```python
from build123d import *

# Parameters (mm, degrees)
SKETCH1_W                      = 50
SKETCH1_H                      = 35
SKETCH1_R                      = 8.5
BOSS_EXTRUDE1_DEPTH            = 8
F_3_0MM_DOWEL_HOLE1_AT_2_COUNT = 2
F_3_0MM_DOWEL_HOLE1_AT_2_PITCH = 40.311288741
M5X0_8_TAPPED_HOLE1_AT_2_COUNT = 2
M5X0_8_TAPPED_HOLE1_AT_2_PITCH = 40.311288741
SKETCH6_R                      = 11.5
CUT_EXTRUDE1_DEPTH             = 1.5
CHAMFER1_SIZE                  = 1
CHAMFER2_SIZE                  = 0.2


with BuildPart() as part:
    # Sketch1 → Boss-Extrude1 (new body)
    with BuildSketch(Plane(origin=(0, 0, 0), x_dir=(1, 0, 0), z_dir=(0, 1, 0))):
        Rectangle(SKETCH1_W, SKETCH1_H)
        with Locations(Location((0, 0, 0), (0, 0, 270))):
            Circle(SKETCH1_R, mode=Mode.SUBTRACT)
    extrude(amount=BOSS_EXTRUDE1_DEPTH)

    # Sketch3 → Ø3.0mm Dowel Hole1 (revolve, cut)
    with BuildSketch(Plane(origin=(-17.5, 8, -10), x_dir=(0, 0, 1), z_dir=(1, 0, 0))):
        Polygon((0, 0), (0, 8), (1.75, 8), (1.5, 7.75), (1.5, 0.25), (1.75, 0), align=None)
    f_3_0mm_dowel_hole1 = revolve(axis=Axis((-17.5, 14.35, -10), (0, -1, 0)), mode=Mode.SUBTRACT)

    # Ø3.0mm Dowel Hole1 at 2: Ø3.0mm Dowel Hole1 ×2
    with Locations(*[Vector(0.8682431421244593, 0, 0.49613893835683387) * (i * F_3_0MM_DOWEL_HOLE1_AT_2_PITCH) for i in range(1, F_3_0MM_DOWEL_HOLE1_AT_2_COUNT)]):
        add(f_3_0mm_dowel_hole1, mode=Mode.SUBTRACT)

    # Sketch5 → M5x0.8 Tapped Hole1 (revolve, cut)
    with BuildSketch(Plane(origin=(17.5, 8, -10), x_dir=(0, 0, 1), z_dir=(1, 0, 0))):
        Polygon((0, 0), (0, 8), (3, 8), (2.1, 7.1), (2.1, 0.9), (3, 0), align=None)
    m5x0_8_tapped_hole1 = revolve(axis=Axis((17.5, 14.35, -10), (0, -1, 0)), mode=Mode.SUBTRACT)

    # M5x0.8 Tapped Hole1 at 2: M5x0.8 Tapped Hole1 ×2
    with Locations(*[Vector(-0.8682431421244593, 0, 0.49613893835683387) * (i * M5X0_8_TAPPED_HOLE1_AT_2_PITCH) for i in range(1, M5X0_8_TAPPED_HOLE1_AT_2_COUNT)]):
        add(m5x0_8_tapped_hole1, mode=Mode.SUBTRACT)

    # Sketch6 → Cut-Extrude1 (cut)
    with BuildSketch(Plane(origin=(0, 8, 0), x_dir=(1, 0, 0), z_dir=(0, 1, 0))):
        with Locations(Location((0, 0, 0), (0, 0, 270))):
            Circle(SKETCH6_R)
    extrude(amount=-CUT_EXTRUDE1_DEPTH, mode=Mode.SUBTRACT)

    # Chamfer1
    chamfer1_edges = [part.edges().sort_by_distance(p)[0] for p in [
        (-25, 4, -17.5),
        (25, 4, -17.5),
        (25, 4, 17.5),
        (-25, 4, 17.5),
    ]]
    chamfer(chamfer1_edges, length=CHAMFER1_SIZE)

    # Chamfer2
    chamfer2_edges = [part.edges().sort_by_distance(p)[0] for p in [
        (0, 0, -8.5),
        (0, 6.5, -8.5),
        (0, 8, -11.5),
        (0, 0, -17.5),
        (0, 8, -17.5),
        (-25, 0, 0),
        (25, 0, 0),
        (0, 0, 17.5),
        (-24.5, 0, 17),
        (-24.5, 0, -17),
        (24.5, 0, 17),
        (24.5, 0, -17),
        (25, 8, 0),
        (-25, 8, 0),
        (0, 8, 17.5),
        (-24.5, 8, 17),
        (-24.5, 8, -17),
        (24.5, 8, 17),
        (24.5, 8, -17),
    ]]
    chamfer(chamfer2_edges, length=CHAMFER2_SIZE)


solid = part.part
```
Geometry: final body of the model. Coordinates: model frame, mm. A direction names the side the tool comes from. Give positions to 0.01 mm unless a question says otherwise; leave off trailing zeros. Write each loop counter-clockwise with the first axis right and the second up, starting at its lowest first coordinate (ties: lowest second). Pieces come first, ordered by that corner, then holes.
1. Section query C-C, the plane y = 2.5. Return loops of the section in (x, z), then the cut area to 3 significant figures.
2. Section query B-B, the plane z = 0. Return loops of the section in (x, y), then the cut area to 3 significant figures.
3. Reachability of faces 1 (the cylindrical face through (8.428, 3.207, -1.107)), 2 (the flat face through (9, 6.5, -2)) from +Z, -Z, +X, -X, +Y, -Y: full face, straight path, thin tool, end or side. Return the list, or none.
4. Pin query (flat end, axial travel): P1, Ø18.5, axis at x = 0, z = 0, coming from the +Y side; P2, Ø18.5, axis at x = 5, z = 0, coming from the +Y side. Return the tip coordinate at first contact, or that it passes through.
5. Section query D-D, the plane x = 17.5. Return loops of the section in (y, z).
6. Line query: probe 1 along Z at (x, y) = (17.5, 5.5); probe 2 along X at (y, z) = (4.75, 10); probe 3 along X at (y, z) = (3, -10). Output: solid intervals per line, ascending.
7. Draft query along X for faces 3 (the flat face through (0, 4, -17.5)), 4 (the cylindrical face through (-18.51, 4.05, -11.11)), 5 (the flat face through (-24.5, 3.9, -17)). Return one class per face: released by +X, released by -X, zero draft, split by the parting line, or undercut.
8. Section query A-A, the plane x = 0. Return loops of the section in (y, z).
Computed:
1. outline: (-25, -16.5) - (-24, -17.5) - (24, -17.5) - (25, -16.5) - (25, 16.5) - (24, 17.5) - (-24, 17.5) - (-25, 16.5) - close; hole circle Ø4.2 at (-17.5, 10); hole circle Ø3 at (-17.5, -10); hole circle Ø17 at (0, 0); hole circle Ø4.2 at (17.5, -10); hole circle Ø3 at (17.5, 10)
1. area: 1,480 mm2
2. outline: (-25, 0.2) - (-24.8, 0) - (-8.7, 0) - (-8.5, 0.2) - (-8.5, 6.3) - (-8.7, 6.5) - (-11.5, 6.5) - (-11.5, 7.8) - (-11.7, 8) - (-24.8, 8) - (-25, 7.8) - close; (8.5, 0.2) - (8.7, 0) - (24.8, 0) - (25, 0.2) - (25, 7.8) - (24.8, 8) - (11.7, 8) - (11.5, 7.8) - (11.5, 6.5) - (8.7, 6.5) - (8.5, 6.3) - close
2. area: 255 mm2
3. face 1: +Y, -Y
3. face 2: +Y
4. P1: stops at y = 6.5
4. P2: stops at y = 8
5. outline: (0, -17.3) - (0.2, -17.5) - (7.8, -17.5) - (8, -17.3) - (8, -13) - (7.1, -12.1) - (0.9, -12.1) - (0, -13) - close; (0, -7) - (0.9, -7.9) - (7.1, -7.9) - (8, -7) - (8, 8.25) - (7.75, 8.5) - (0.25, 8.5) - (0, 8.25) - close; (0, 11.75) - (0.25, 11.5) - (7.75, 11.5) - (8, 11.75) - (8, 17.3) - (7.8, 17.5) - (0.2, 17.5) - (0, 17.3) - close
6. probe 1: z = -17.5 to -12.1, -7.9 to 8.5, 11.5 to 17.5
6. probe 2: x = -25 to -19.6, -15.4 to 16, 19 to 25
6. probe 3: x = -25 to -19, -16 to 15.4, 19.6 to 25
7. face 3: zero draft
7. face 4: undercut
7. face 5: released by -X
8. outline: (0, -17.3) - (0.2, -17.5) - (7.8, -17.5) - (8, -17.3) - (8, -11.7) - (7.8, -11.5) - (6.5, -11.5) - (6.5, -8.7) - (6.3, -8.5) - (0.2, -8.5) - (0, -8.7) - close; (0, 8.7) - (0.2, 8.5) - (6.3, 8.5) - (6.5, 8.7) - (6.5, 11.5) - (7.8, 11.5) - (8, 11.7) - (8, 17.3) - (7.8, 17.5) - (0.2, 17.5) - (0, 17.3) - close
